For this review, take the finished solid that the model builds, in its own axes (mm). A direction names the side the tool comes from. Give positions to 0.01 mm unless a question says otherwise; leave off trailing zeros. Write each loop counter-clockwise with the first axis right and the second up, starting at its lowest first coordinate (ties: lowest second). Pieces come first, ordered by that corner, then holes. Notation, with made-up numbers: M -38,-34.75 L -31,-34.75 A13 ccw -31,-13.75 Z; hole C 0,39.5 d11. An arc over 180 degrees is marked long. Use one line per item in the form item = value. Start each with the question number.
Q1. For probe 1 along Z at (x, y) = (-6, 7); probe 2 along Z at (x, y) = (26.5, 7.25); probe 3 along X at (y, z) = (5, -49), list the stretches that pass through material, from the lowest coordinate up. Write a range as [from, to].
Q2. Consider section A-A on y = 5. Write out the cut boundary in (x, z).
Q3. Consider section D-D on z = -38.5. Write out the cut boundary in (x, y), and give its area (3 significant figures).
Q4. Consider section B-B on z = -61.5. Write out the cut boundary in (x, y), and give its area (3 significant figures).
Q5. Consider section C-C on x = -31. Write out the cut boundary in (y, z).
Q6. Mouldability with a two-part tool opening along Z and no side actions: class faces 6 (the flat face through (4.2, 1.8, -60.658)), 7 (the cylindrical face through (1.08, 0.12, -50.52)), 8 (the flat face through (0, 5, -65.658)), 9 (the flat face through (-3.06, -0.41, -63.12)) as released by +Z, released by -Z, zero draft, split by the parting line, or undercut.
Q7. Clearance check with flat-ended pins moving along their axes: pin 1 Ø5.5 at (y, z) = (6.5, -63) entering from +X; pin 2 Ø2 at (x, y) = (-6, 9.5) entering from -Z; pin 3 Ø1.5 at (y, z) = (6, -62.5) entering from -X; pin 4 Ø8 at (x, y) = (16, 3.5) entering from -Z. State where each tip first meets the part, or that it passes through.
Q8. Tool access review of faces 1 (the flat face through (6.215, 5, -63)), 2 (the flat face through (-6.215, 5, -63)), 3 (the flat face through (3.06, 10.41, -63.12)), 4 (the flat face through (3.151, -0.357, -63.123)), 5 (the flat face through (-3.151, 10.357, -63.123)): name each direction out of +Z, -Z, +X, -X, +Y, -Y from which nothing blocks a thin tool from reaching the whole face with its end or side.
```python
from build123d import *

# Parameters (mm, degrees)
BOSS_EXTRUDE1_DEPTH = 10
SKETCH2_R           = 5
BOSS_EXTRUDE2_DEPTH = 20
BOSS_EXTRUDE4_DEPTH = 5


with BuildPart() as part:
    # Sketch1 → Boss-Extrude1 (new body)
    with BuildSketch(Plane(origin=(0, 0, 0), x_dir=(1, 0, 0), z_dir=(0, 1, 0))):
        Polygon((-35, 40.657635654), (0, 40.657635654), (35, 40.657635654), (35, 0.657635654), (-35, 0.657635654), align=None)
    extrude(amount=BOSS_EXTRUDE1_DEPTH)

    # Sketch2 → Boss-Extrude2 (add)
    with BuildSketch(Plane(origin=(0, 0, -40.657635654), x_dir=(-1, 0, 0), z_dir=(0, 0, -1))):
        with Locations((0, 5)):
            Circle(SKETCH2_R)
    extrude(amount=BOSS_EXTRUDE2_DEPTH)

    # Sketch3 → Boss-Extrude4 (add)
    with BuildSketch(Plane(origin=(0, 0, -60.657635654), x_dir=(-1, 0, 0), z_dir=(0, 0, -1))):
        Polygon((0, -2.176119405), (6.214701705, 1.411940298), (6.214701705, 8.588059702), (0, 12.176119405), (-6.214701705, 8.588059702), (-6.214701705, 1.411940298), align=None)
    extrude(amount=BOSS_EXTRUDE4_DEPTH)


solid = part.part
```
Working result:
q1.probe_1 = [-65.66, -60.66], [-40.66, -0.66]
q1.probe_2 = [-40.66, -0.66]
q1.probe_3 = [-5, 5]
q2.outline = M -35,-40.66 L -5,-40.66 L -5,-60.66 L -6.21,-60.66 L -6.21,-65.66 L 6.21,-65.66 L 6.21,-60.66 L 5,-60.66 L 5,-40.66 L 35,-40.66 L 35,-0.66 L -35,-0.66 Z
q3.outline = M -35,0 L 35,0 L 35,10 L -35,10 Z
q3.area = 700 mm²
q4.outline = M -6.21,1.41 L 0,-2.18 L 6.21,1.41 L 6.21,8.59 L 0,12.18 L -6.21,8.59 Z
q4.area = 134 mm²
q5.outline = M 0,-40.66 L 10,-40.66 L 10,-0.66 L 0,-0.66 Z
q6.face_6 = undercut
q6.face_7 = undercut
q6.face_8 = released by -Z
q6.face_9 = zero draft
q7.pin_1 = 6.21
q7.pin_2 = -65.66
q7.pin_3 = -6.21
q7.pin_4 = -40.66
q8.face_1 = -Z, +X, +Y, -Y
q8.face_2 = -Z, -X, +Y, -Y
q8.face_3 = -Z, +X, +Y
q8.face_4 = -Z, +X, -Y
q8.face_5 = -Z, -X, +Y
